Model file for the job. Use its own axes, mm. Face numbers are marked on the shaded views. A direction names the side the tool comes from. Round coordinates to 2 decimals unless told otherwise and drop trailing zeros. Loops run counter-clockwise (first coordinate to the right, second up) from the corner with the lowest first, then second, coordinate; pieces in that order, holes last. Notation, with made-up numbers: M 28,48.25 L 45,48.25 A11 ccw 45,62.25 Z; hole C 65,5.25 d4. An arc over 180 degrees is marked long. Answer in a Markdown table with one row per item.
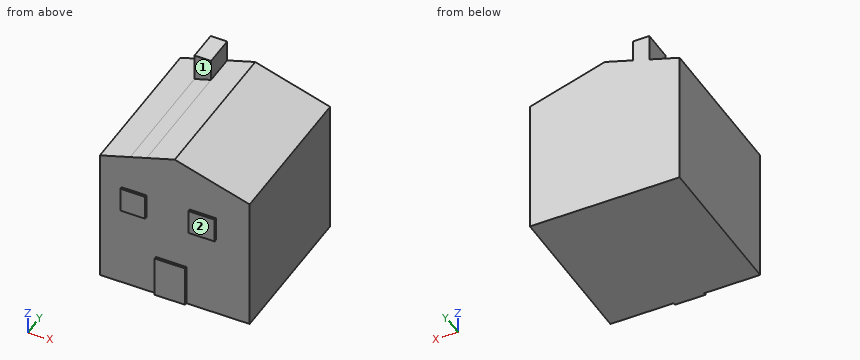
from build123d import *

# Parameters (mm, degrees)
F0_W     = 122.8438019753
F0_H     = 112.1096983552
F1_DEPTH = 127
F2_DEPTH = 25.4
F3_W     = 24.9869422987
F3_H     = 34.055031836
F4_DEPTH = 2
F5_W     = 10.221931152
F5_H     = 10.2219306864
F5_W_2   = 21.4697401971
F5_H_2   = 20.4438613728
F6_DEPTH = 2


with BuildPart() as f1:
    # F0 (on Front) → F1 (new body)
    with BuildSketch(Plane.XZ):
        Rectangle(F0_W, F0_H)
        Polygon((-61.4219009876, 56.0548491776), (61.4219009876, 56.0548491776), (0, 75.0973075628), (-23.0313282844, 67.9569699412), (-36.6085842252, 63.7476516512), align=None)
    extrude(amount=F1_DEPTH)

    # F0 (on Front) → F2 (join)
    with BuildSketch(Plane.XZ):
        Polygon((-36.6085842252, 85.7438147068), (-36.6085842252, 63.7476516512), (-23.0313282844, 67.9569699412), (-23.0313282844, 85.7438147068), align=None)
    extrude(amount=F2_DEPTH)

    # F3 (on face) → F4 (join)
    with BuildSketch(Plane.XZ.offset(127)):
        with Locations((-2.9205507599, -39.0273332596)):
            Rectangle(F3_W, F3_H)
    extrude(amount=F4_DEPTH)

    # F5 (on face) → F6 (join)
    with BuildSketch(Plane.XZ.offset(127)):
        with Locations((-38.5350571014, 27.7306872886)):
            Rectangle(F5_W, F5_H)
        with Locations((-28.3131259494, 27.7306872886)):
            Rectangle(F5_W, F5_H)
        with Locations((-38.5350571014, 17.5087566022)):
            Rectangle(F5_W, F5_H)
        with Locations((-28.3131259494, 17.5087566022)):
            Rectangle(F5_W, F5_H)
        with Locations((22.9804925621, 22.6197219454)):
            Rectangle(F5_W_2, F5_H_2)
    extrude(amount=F6_DEPTH)


solid = f1.part
1. Saw through at C-C (z = 50.5). Write the cut outline in (x, y), and give its area (3 significant figures).
Verdict:
| item | result |
|---|---|
| outline | M -61.42,-127 L 61.42,-127 L 61.42,0 L -61.42,0 Z |
| area | 15,600 mm² |
2. Tool access for the marked faces 1 and 2: list every direction of +Z, -Z, +X, -X, +Y, -Y with a clear straight run to the whole face (end or side of a thin tool).
Verdict:
| item | result |
|---|---|
| face 1 | +Z, -X, -Y |
| face 2 | +Z, -Z, +X, -X, -Y |
3. Wall check: probe 1 along Y at (x, z) = (-2.5, -17); probe 2 along Z at (x, y) = (-8.5, -4.5); probe 3 along Z at (x, y) = (42, -60). Give the ranges that are in metal, low to high.
Verdict:
| item | result |
|---|---|
| probe 1 | y = -127 to 0 |
| probe 2 | z = -56.05 to 72.46 |
| probe 3 | z = -56.05 to 62.08 |
4. Saw through at B-B (x = -6). Write the cut outline in (y, z).
Verdict:
| item | result |
|---|---|
| outline | M -129,-56.05 L 0,-56.05 L 0,73.24 L -127,73.24 L -127,-22 L -129,-22 Z |
5. Saw through at D-D (y = -97). Write the cut outline in (x, z), and give its area (3 significant figures).
Verdict:
| item | result |
|---|---|
| outline | M -61.42,-56.05 L 61.42,-56.05 L 61.42,56.05 L 0,75.1 L -61.42,56.05 Z |
| area | 14,900 mm² |
6. Saw through at A-A (y = -18). Write the cut outline in (x, z), and give its area (3 significant figures).
Verdict:
| item | result |
|---|---|
| outline | M -61.42,-56.05 L 61.42,-56.05 L 61.42,56.05 L 0,75.1 L -23.03,67.96 L -23.03,85.74 L -36.61,85.74 L -36.61,63.75 L -61.42,56.05 Z |
| area | 15,200 mm² |
7. Pin check, flat tips, straight feed: pin 1 (2 mm diameter, centred on x = -5, y = -127.5, fed in from +Z); pin 2 (0.6 mm diameter, centred on y = -128, z = 18, fed in from -X); pin 3 (1 mm diameter, centred on x = 24.5, z = -14.5, fed in from -Y); pin 4 (3 mm diameter, centred on x = 13.5, z = 50.5, fed in from +Y). Stop position of each tip, or through.
Verdict:
| item | result |
|---|---|
| pin 1 | stops at z = 73.82 |
| pin 2 | stops at x = -43.65 |
| pin 3 | stops at y = -127 |
| pin 4 | stops at y = 0 |
